Work out the finished part from the listing and answer in its coordinate system (mm). Face numbers are marked on the shaded views. A direction names the side the tool comes from. Round coordinates to 2 decimals unless told otherwise and drop trailing zeros. Order: outer loops, then holes, each group sorted by start corner. A loop starts at its lowest first (then second) coordinate and runs counter-clockwise, first axis right, second up.
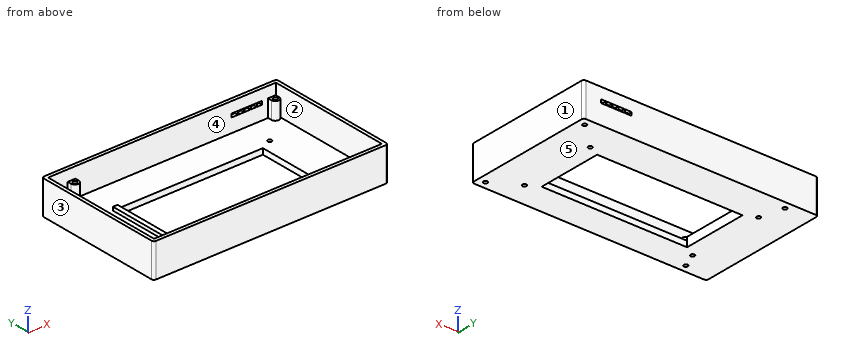
from build123d import *

# Parameters (mm, degrees)
F0_W      = 205
F0_H      = 115
F1_DEPTH  = 5
F2_R      = 1.75
F3_DEPTH  = 25
F4_W      = 127
F4_H      = 57
F5_DEPTH  = 25
F7_DEPTH  = 15
F9_DEPTH  = 3
F10_W     = 4
F10_H     = 57
F11_DEPTH = 3
F12_R     = 1.75
F13_DEPTH = 25
F14_R     = 1.75
F15_DEPTH = 25
F16_R     = 1.75
F17_DEPTH = 25
F18_R     = 1.75
F19_DEPTH = 25
F20_R     = 1.75
F21_DEPTH = 5
F22_W     = 168.3
F22_H     = 3
F23_DEPTH = 24.5
F24_R     = 2
F25_W     = 27
F25_H     = 3
F26_DEPTH = 25
F27_W     = 0.4
F27_H     = 3
F28_DEPTH = 3
F29_W     = 6.7
F29_H     = 3
F30_DEPTH = 9.5
F31_W     = 6.7
F31_H     = 3
F32_DEPTH = 9.5
F33_W     = 6.7
F33_H     = 3
F34_DEPTH = 9.5
F35_W     = 6.7
F35_H     = 3
F36_DEPTH = 9.5


# Not quite as in the source:
# - a feature names something its author has since deleted; it is built from what else it names


with BuildPart() as f1:
    # F0 (on Top) → F1 (new body)
    with BuildSketch(Plane.XY):
        with Locations((0.1253969967, -22.0995221115)):
            Rectangle(F0_W, F0_H)
    extrude(amount=F1_DEPTH)

    # F2 (on face) → F3 (cut)
    with BuildSketch(Plane(origin=(0, 0, 0), x_dir=(1, 0, 0), z_dir=(0, 0, -1))):
        with Locations((-73.3746030033, 59.5995221115)):
            Circle(F2_R)
        with Locations((-73.3746030033, -8.1444778885)):
            Circle(F2_R)
        with Locations((73.6253969967, 59.5995221115)):
            Circle(F2_R)
        with Locations((73.6253969967, -8.1444778885)):
            Circle(F2_R)
    extrude(amount=-F3_DEPTH, mode=Mode.SUBTRACT)

    # F4 (on face) → F5 (cut)
    with BuildSketch(Plane(origin=(0, 0, 0), x_dir=(1, 0, 0), z_dir=(0, 0, -1))):
        with Locations((0.1253969967, 25.0995221115)):
            Rectangle(F4_W, F4_H)
    extrude(amount=-F5_DEPTH, mode=Mode.SUBTRACT)

    # F6 (on face) → F7 (join)
    with BuildSketch(Plane.XY.offset(5)):
        with BuildLine():
            Line((96.1253969967, -73.0995221115), (99.4753969967, -73.0995221115))
            ThreePointArc((99.4753969967, -73.0995221115), (96.1253969967, -69.7495221115), (92.7753969967, -73.0995221115))
            Line((92.7753969967, -73.0995221115), (96.1253969967, -73.0995221115))
        make_face()
        with BuildLine():
            ThreePointArc((92.7753969967, -73.0995221115), (96.1253969967, -76.4495221115), (99.4753969967, -73.0995221115))
            Line((99.4753969967, -73.0995221115), (96.1253969967, -73.0995221115))
            Line((96.1253969967, -73.0995221115), (92.7753969967, -73.0995221115))
        make_face()
        with BuildLine():
            Line((-78.8746030033, -73.0995221115), (-75.5246030033, -73.0995221115))
            ThreePointArc((-75.5246030033, -73.0995221115), (-78.8746030033, -69.7495221115), (-82.2246030033, -73.0995221115))
            Line((-82.2246030033, -73.0995221115), (-78.8746030033, -73.0995221115))
        make_face()
        with BuildLine():
            ThreePointArc((-82.2246030033, -73.0995221115), (-78.8746030033, -76.4495221115), (-75.5246030033, -73.0995221115))
            Line((-75.5246030033, -73.0995221115), (-78.8746030033, -73.0995221115))
            Line((-78.8746030033, -73.0995221115), (-82.2246030033, -73.0995221115))
        make_face()
        with BuildLine():
            Line((96.1253969967, 28.9004778885), (99.4753969967, 28.9004778885))
            ThreePointArc((99.4753969967, 28.9004778885), (96.1253969967, 32.2504778885), (92.7753969967, 28.9004778885))
            Line((92.7753969967, 28.9004778885), (96.1253969967, 28.9004778885))
        make_face()
        with BuildLine():
            ThreePointArc((92.7753969967, 28.9004778885), (96.1253969967, 25.5504778885), (99.4753969967, 28.9004778885))
            Line((99.4753969967, 28.9004778885), (96.1253969967, 28.9004778885))
            Line((96.1253969967, 28.9004778885), (92.7753969967, 28.9004778885))
        make_face()
        with BuildLine():
            ThreePointArc((-82.2246030033, 28.9004778885), (-78.8746030033, 25.5504778885), (-75.5246030033, 28.9004778885))
            ThreePointArc((-75.5246030033, 28.9004778885), (-78.8746030033, 32.2504778885), (-82.2246030033, 28.9004778885))
        make_face()
        with BuildLine():
            Line((-82.2246030033, -79.5995221115), (-75.5246030033, -79.5995221115))
            Line((-75.5246030033, -79.5995221115), (-75.5246030033, -73.0995221115))
            ThreePointArc((-75.5246030033, -73.0995221115), (-78.8746030033, -76.4495221115), (-82.2246030033, -73.0995221115))
            Line((-82.2246030033, -73.0995221115), (-82.2246030033, -79.5995221115))
        make_face()
        with BuildLine():
            Line((-75.5246030033, 28.9004778885), (-75.5246030033, 35.4004778885))
            Line((-75.5246030033, 35.4004778885), (-82.2246030033, 35.4004778885))
            Line((-82.2246030033, 35.4004778885), (-82.2246030033, 28.9004778885))
            ThreePointArc((-82.2246030033, 28.9004778885), (-78.8746030033, 32.2504778885), (-75.5246030033, 28.9004778885))
        make_face()
        with BuildLine():
            Line((99.4753969967, 28.9004778885), (99.4753969967, 35.4004778885))
            Line((99.4753969967, 35.4004778885), (92.7753969967, 35.4004778885))
            Line((92.7753969967, 35.4004778885), (92.7753969967, 28.9004778885))
            ThreePointArc((92.7753969967, 28.9004778885), (96.1253969967, 32.2504778885), (99.4753969967, 28.9004778885))
        make_face()
        with BuildLine():
            Line((99.4753969967, -79.5995221115), (99.4753969967, -73.0995221115))
            ThreePointArc((99.4753969967, -73.0995221115), (96.1253969967, -76.4495221115), (92.7753969967, -73.0995221115))
            Line((92.7753969967, -73.0995221115), (92.7753969967, -79.5995221115))
            Line((92.7753969967, -79.5995221115), (99.4753969967, -79.5995221115))
        make_face()
    extrude(amount=F7_DEPTH)

    # F8 (on face) → F9 (join)
    with BuildSketch(Plane.XY.offset(5)):
        with BuildLine():
            ThreePointArc((-92.3746030033, -23.0995221115), (-88.8746030033, -26.5995221115), (-85.3746030033, -23.0995221115))
            Line((-85.3746030033, -23.0995221115), (-92.3746030033, -23.0995221115))
        make_face()
        with BuildLine():
            Line((-92.3746030033, -23.0995221115), (-85.3746030033, -23.0995221115))
            ThreePointArc((-85.3746030033, -23.0995221115), (-88.8746030033, -19.5995221115), (-92.3746030033, -23.0995221115))
        make_face()
    extrude(amount=F9_DEPTH)

    # F10 (on face) → F11 (join)
    with BuildSketch(Plane.XY.offset(5)):
        with Locations((-65.3746030033, -25.0995221115)):
            Rectangle(F10_W, F10_H)
    extrude(amount=F11_DEPTH)

    # F12 (on face) → F13 (cut)
    with BuildSketch(Plane.XY.offset(20)):
        with Locations((-78.8746030033, -73.0995221115)):
            Circle(F12_R)
    extrude(amount=-F13_DEPTH, mode=Mode.SUBTRACT)

    # F14 (on face) → F15 (cut)
    with BuildSketch(Plane.XY.offset(20)):
        with Locations((-78.8746030033, 28.9004778885)):
            Circle(F14_R)
    extrude(amount=-F15_DEPTH, mode=Mode.SUBTRACT)

    # F16 (on face) → F17 (cut)
    with BuildSketch(Plane.XY.offset(20)):
        with Locations((96.1253969967, -73.0995221115)):
            Circle(F16_R)
    extrude(amount=-F17_DEPTH, mode=Mode.SUBTRACT)

    # F18 (on face) → F19 (cut)
    with BuildSketch(Plane.XY.offset(20)):
        with Locations((96.1253969967, 28.9004778885)):
            Circle(F18_R)
    extrude(amount=-F19_DEPTH, mode=Mode.SUBTRACT)

    # F20 (on face) → F21 (cut)
    with BuildSketch(Plane.XY.offset(8)):
        with Locations((-88.8746030033, -23.0995221115)):
            Circle(F20_R)
    extrude(amount=-F21_DEPTH, mode=Mode.SUBTRACT)

    # F22 (on face) → F23 (join)
    with BuildSketch(Plane.XY.offset(5)):
        Polygon((99.4753969967, -79.5995221115), (102.6253969967, -79.5995221115), (102.6253969967, 35.4004778885), (99.4753969967, 35.4004778885), (99.4753969967, 32.4004778885), (99.6253969967, 32.4004778885), (99.6253969967, -76.5995221115), (99.4753969967, -76.5995221115), align=None)
        Polygon((-102.3746030033, -79.5995221115), (-82.2246030033, -79.5995221115), (-82.2246030033, -76.5995221115), (-99.3746030033, -76.5995221115), (-99.3746030033, 32.4004778885), (-82.2246030033, 32.4004778885), (-82.2246030033, 35.4004778885), (-102.3746030033, 35.4004778885), align=None)
        with Locations((8.6253969967, -78.0995221115)):
            Rectangle(F22_W, F22_H)
        with Locations((8.6253969967, 33.9004778885)):
            Rectangle(F22_W, F22_H)
    extrude(amount=F23_DEPTH)

    # F24
    f24_edges = [f1.edges().sort_by_distance(p)[0] for p in [
        (-102.374603, -79.599522, 14.75),
        (102.625397, -79.599522, 14.75),
        (102.625397, 35.400478, 14.75),
        (-102.374603, 35.400478, 14.75),
    ]]
    fillet(f24_edges, radius=F24_R)

    # F25 (on face) → F26 (cut)
    with BuildSketch(Plane.XZ.offset(-32.4004778885)):
        with Locations((74.1253969967, 18.5)):
            Rectangle(F25_W, F25_H)
    extrude(amount=-F26_DEPTH, mode=Mode.SUBTRACT)

    # F27 (on face) → F28 (join)
    with BuildSketch(Plane.XY.offset(17)):
        with Locations((82.9253969967, 33.9004778885)):
            Rectangle(F27_W, F27_H)
        with Locations((77.5253969967, 33.9004778885)):
            Rectangle(F27_W, F27_H)
        with Locations((72.1253969967, 33.9004778885)):
            Rectangle(F27_W, F27_H)
        with Locations((66.7253969967, 33.9004778885)):
            Rectangle(F27_W, F27_H)
    extrude(amount=F28_DEPTH)

    # F29 (on face) → F30 (join)
    with BuildSketch(Plane.XY.offset(20)):
        with Locations((-78.8746030033, -78.0995221115)):
            Rectangle(F29_W, F29_H)
    extrude(amount=F30_DEPTH)

    # F31 (on face) → F32 (join)
    with BuildSketch(Plane.XY.offset(20)):
        with Locations((96.1253969967, -78.0995221115)):
            Rectangle(F31_W, F31_H)
    extrude(amount=F32_DEPTH)

    # F33 (on face) → F34 (join)
    with BuildSketch(Plane.XY.offset(20)):
        with Locations((96.1253969967, 33.9004778885)):
            Rectangle(F33_W, F33_H)
    extrude(amount=F34_DEPTH)

    # F35 (on face) → F36 (join)
    with BuildSketch(Plane.XY.offset(20)):
        with Locations((-78.8746030033, 33.9004778885)):
            Rectangle(F35_W, F35_H)
    extrude(amount=F36_DEPTH)


solid = f1.part
Item 1: Find section A-A (y = -51). Write down the section's boundary in (x, z), plus the area to 3 significant figures.
Item 2: Find section D-D (z = 10). State how many separate pieces and enclosed holes the cut face has, plus the area to 3 significant figures.
Item 3: Find section B-B (z = 22.75). Write down the section's boundary in (x, y).
Item 4: Find section C-C (x = -16). Write down the section's boundary in (y, z).
Item 5: For a pull along X with two mould halves and no side action, classify the marked faces 3, 4 and 5 as released by +X, released by -X, zero draft, split by the parting line, or undercut.
Item 6: Given pin 1 (4.5 mm diameter, centred on x = -73.37, y = -59.6, fed in from +Z), flat-ended and moving along its own axis, determine where the tip first touches the part or whether it passes through.
Item 7: A tool of negligible diameter and unlimited length cuts with its end or side. For the marked faces 1 and 2, from which of +Z, -Z, +X, -X, +Y, -Y can it reach the whole face along a straight path? Write none if from no direction.
Item 8: Find the intervals of material crossed by line 1 along Y through (x, z) = (85, 9.25); line 2 along X through (y, z) = (-29, 7.75); line 3 along X through (y, z) = (-74, 19.75), in increasing order.
Model answer:
1. outline: (-102.37, 0) - (-63.37, 0) - (-63.37, 8) - (-67.37, 8) - (-67.37, 5) - (-99.37, 5) - (-99.37, 29.5) - (-102.37, 29.5) - close; (63.63, 0) - (102.63, 0) - (102.63, 29.5) - (99.63, 29.5) - (99.63, 5) - (63.63, 5) - close
1. area: 549 mm2
2. separate pieces: 1
2. enclosed holes: 5
2. area: 2,010 mm2
3. outline: (-102.37, -77.6) arc R2 ccw to (-100.37, -79.6) - (100.63, -79.6) arc R2 ccw to (102.63, -77.6) - (102.63, 33.4) arc R2 ccw to (100.63, 35.4) - (-100.37, 35.4) arc R2 ccw to (-102.37, 33.4) - close; hole (-99.37, -76.6) - (99.63, -76.6) - (99.63, 32.4) - (-99.37, 32.4) - close
4. outline: (-79.6, 0) - (-53.6, 0) - (-53.6, 5) - (-76.6, 5) - (-76.6, 29.5) - (-79.6, 29.5) - close; (3.4, 0) - (35.4, 0) - (35.4, 29.5) - (32.4, 29.5) - (32.4, 5) - (3.4, 5) - close
5. face 3: released by -X
5. face 4: undercut
5. face 5: zero draft
6. pin 1: stops at z = 5
7. face 1: +Z, -Z, +X, +Y, -Y
7. face 2: +Z
8. line 1: y = -79.6 to -76.6, 32.4 to 35.4
8. line 2: x = -102.37 to -99.37, -67.37 to -63.37, 99.63 to 102.63
8. line 3: x = -102.37 to -99.37, -82.22 to -80.38, -77.37 to -75.52, 92.78 to 94.62, 97.63 to 99.48, 99.63 to 102.63
